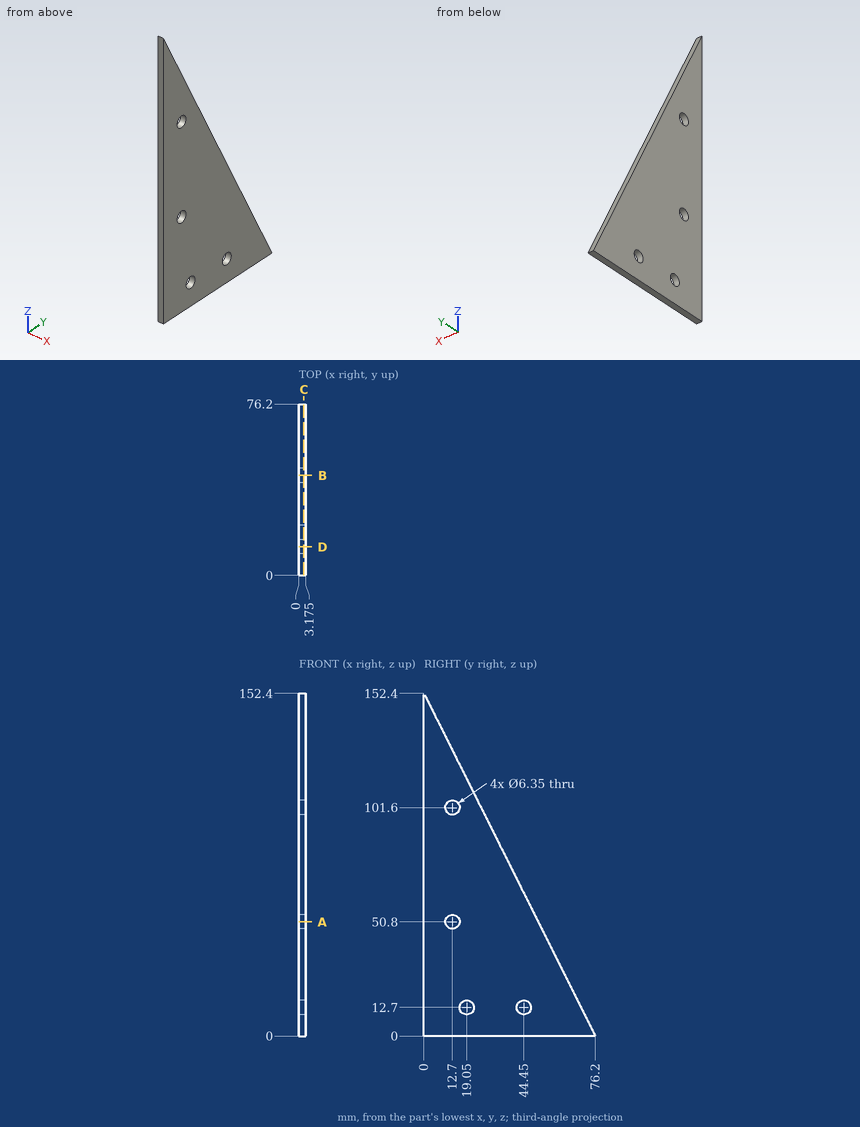
Check sheet for the drawn part. Datum: minimum x, y, z corner. Units: mm. Round coordinates to 2 decimals unless told otherwise and drop trailing zeros. Write each loop counter-clockwise with the first axis right and the second up, starting at its lowest first coordinate (ties: lowest second). Pieces come first, ordered by that corner, then holes. Notation, with made-up numbers: (29, 25.25) -> (45, 25.25) arc R15 cw to (45, 42.25) -> close; hole circle Ø7 at (34, -33.5). An arc over 180 degrees is marked (long way). Put each result on its own line as item: value.
(1) Sectioned sample at D-D (y = 12.7). Enter the section's corners in (x, z) (3 decimals).
Values found:
outline: (0, 0) -> (3.175, 0) -> (3.175, 47.625) -> (0, 47.625) -> close; (0, 53.975) -> (3.175, 53.975) -> (3.175, 98.425) -> (0, 98.425) -> close; (0, 104.775) -> (3.175, 104.775) -> (3.175, 127) -> (0, 127) -> close
(2) Sectioned sample at A-A (z = 50.8). Enter the section's corners in (x, y) (3 decimals).
Values found:
outline: (0, 0) -> (3.175, 0) -> (3.175, 9.525) -> (0, 9.525) -> close; (0, 15.875) -> (3.175, 15.875) -> (3.175, 50.8) -> (0, 50.8) -> close
(3) Sectioned sample at C-C (x = 2.25). Enter the section's corners in (y, z) (3 decimals).
Values found:
outline: (0, 0) -> (76.2, 0) -> (0, 152.4) -> close; hole circle Ø6.35 at (12.7, 50.8); hole circle Ø6.35 at (12.7, 101.6); hole circle Ø6.35 at (19.05, 12.7); hole circle Ø6.35 at (44.45, 12.7)
(4) Material ranges on line 1 (Z direction, x = 0.75, y = 12.7) (3 decimals); line 2 (Y direction, x = 0.45, z = 11.5); line 3 (Y direction, x = 1.75, z = 12.7) (3 decimals), recorded low to high.
Values found:
line 1: z = 0 to 47.625, 53.975 to 98.425, 104.775 to 127
line 2: y = 0 to 16.11, 21.99 to 41.51, 47.39 to 70.45
line 3: y = 0 to 15.875, 22.225 to 41.275, 47.625 to 69.85
(5) Sectioned sample at B-B (y = 44.45). Enter the section's corners in (x, z) (3 decimals).
Values found:
outline: (0, 0) -> (3.175, 0) -> (3.175, 9.525) -> (0, 9.525) -> close; (0, 15.875) -> (3.175, 15.875) -> (3.175, 63.5) -> (0, 63.5) -> close
(6) Go/stop test with a flat-tipped pin: pin 1 Ø5 at (y, z) = (12.7, 50.8) entering from +X. Record where the tip stops, or that it passes through.
Values found:
pin 1: passes through
